Check sheet for the modelled part. Datum: model origin and axes. Units: mm. A direction names the side the tool comes from. Round coordinates to 2 decimals unless told otherwise and drop trailing zeros. Order: outer loops, then holes, each group sorted by start corner. A loop starts at its lowest first (then second) coordinate and runs counter-clockwise, first axis right, second up.
from build123d import *

# Parameters (mm, degrees)
SKETCH1_W           = 30.1625
SKETCH1_H           = 14.2875
BOSS_EXTRUDE1_DEPTH = 6.35
SKETCH2_W           = 30.1625
SKETCH2_H           = 7.9375
BOSS_EXTRUDE2_DEPTH = 6.35
BOSS_EXTRUDE3_DEPTH = 1.5875
SKETCH4_R           = 1.5875
CUT_EXTRUDE1_DEPTH  = 1.5875


with BuildPart() as part:
    # Sketch1 → Boss-Extrude1 (new body)
    with BuildSketch(Plane.XY):
        Rectangle(SKETCH1_W, SKETCH1_H)
    extrude(amount=BOSS_EXTRUDE1_DEPTH)

    # Sketch2 → Boss-Extrude2 (add)
    with BuildSketch(Plane.XY.offset(6.35)):
        Rectangle(SKETCH2_W, SKETCH2_H)
    extrude(amount=BOSS_EXTRUDE2_DEPTH)

    # Sketch3 → Boss-Extrude3 (add)
    with BuildSketch(Plane(origin=(0, 0, 0), x_dir=(-1, 0, 0), z_dir=(0, 0, -1))):
        with BuildLine():
            ThreePointArc((-15.08125, 0), (-16.243669962, 2.806330038), (-19.05, 3.96875))
            Line((-19.05, 3.96875), (-19.05, -3.96875))
            ThreePointArc((-19.05, -3.96875), (-16.243669962, -2.806330038), (-15.08125, 0))
        make_face()
        with BuildLine():
            Line((-19.05, -3.96875), (-19.05, 3.96875))
            ThreePointArc((-19.05, 3.96875), (-23.01875, 0), (-19.05, -3.96875))
        make_face()
        with BuildLine():
            Line((-15.08125, 3.96875), (-19.05, 3.96875))
            ThreePointArc((-19.05, 3.96875), (-16.243669962, 2.806330038), (-15.08125, 0))
            Line((-15.08125, 0), (-15.08125, 3.96875))
        make_face()
        with BuildLine():
            ThreePointArc((-15.08125, 0), (-16.243669962, -2.806330038), (-19.05, -3.96875))
            Line((-19.05, -3.96875), (-15.08125, -3.96875))
            Line((-15.08125, -3.96875), (-15.08125, 0))
        make_face()
    boss_extrude3 = extrude(amount=-BOSS_EXTRUDE3_DEPTH)

    # Sketch4 → Cut-Extrude1 (cut)
    with BuildSketch(Plane.XY.offset(1.5875)):
        with Locations((18.966101938, 0)):
            Circle(SKETCH4_R)
    cut_extrude1 = extrude(amount=-CUT_EXTRUDE1_DEPTH, mode=Mode.SUBTRACT)

    # Mirror1: Boss-Extrude3, Cut-Extrude1 across plane
    add(boss_extrude3.mirror(Plane(origin=(0, 0, 0), x_dir=(0, 0, 1), z_dir=(1, 0, 0))))
    add(cut_extrude1.mirror(Plane(origin=(0, 0, 0), x_dir=(0, 0, 1), z_dir=(1, 0, 0))), mode=Mode.SUBTRACT)


solid = part.part
1) Set-up check for faces 5 (the face through (-17, 3.969, 1)), 6 (the face through (0, -3.969, 9)), 7 (the face through (0, 3.969, 9)): record each of +Z, -Z, +X, -X, +Y, -Y from which the full face is reachable in a straight line by a thin tool's end or side.
2) Gauge pin test, flat ends, axial feed: pin 1 (0.8 mm diameter, centred on x = 18, z = 1, fed in from +Y); pin 2 (4 mm diameter, centred on x = -18.97, y = 0, fed in from +Z); pin 3 (1.7 mm diameter, centred on x = 16, z = 0.5, fed in from -Y). Record the tip position at first contact, or that the pin passes through.
3) Sectioned sample at C-C on z = 11.75. Record the cut outline in (x, y), and give its area (3 significant figures).
4) Sectioned sample at B-B on x = 8. Record the cut outline in (y, z), and give its area (3 significant figures).
5) Sectioned sample at D-D on y = -3. Record the cut outline in (x, z).
6) Sectioned sample at A-A on y = 0. Record the cut outline in (x, z).
7) Scan lines: line 1 (Y direction, x = -5, z = 10.75); line 2 (Z direction, x = 19, y = 2.5); line 3 (X direction, y = -5.5, z = 3). Record each from-to range of solid material in increasing order.
8) Draft check along Y on faces 1 (the face through (-17, -3.969, 1)), 2 (the face through (17, 3.969, 1)), 3 (the face through (-17, 0, 1.588)), 4 (the face through (20.48, 0.48, 0.8)). Enter one of: pulls with the +Y half, pulls with the -Y half, needs draft (parallel to the pull), parting line crosses it, or undercut.
Values found:
1. face 5: +Z, -Z, -X, +Y
1. face 6: +Z, +X, -X, -Y
1. face 7: +Z, +X, -X, +Y
2. pin 1: stops at y = 3.97
2. pin 2: stops at z = 1.59
2. pin 3: stops at y = -3.97
3. outline: (-15.08, -3.97) - (15.08, -3.97) - (15.08, 3.97) - (-15.08, 3.97) - close
3. area: 239 mm2
4. outline: (-7.14, 0) - (7.14, 0) - (7.14, 6.35) - (3.97, 6.35) - (3.97, 12.7) - (-3.97, 12.7) - (-3.97, 6.35) - (-7.14, 6.35) - close
4. area: 141 mm2
5. outline: (-21.65, 0) - (21.65, 0) - (21.65, 1.59) - (15.08, 1.59) - (15.08, 12.7) - (-15.08, 12.7) - (-15.08, 1.59) - (-21.65, 1.59) - close
6. outline: (-23.02, 0) - (-20.55, 0) - (-20.55, 1.59) - (-23.02, 1.59) - close; (-17.38, 0) - (17.38, 0) - (17.38, 1.59) - (15.08, 1.59) - (15.08, 12.7) - (-15.08, 12.7) - (-15.08, 1.59) - (-17.38, 1.59) - close; (20.55, 0) - (23.02, 0) - (23.02, 1.59) - (20.55, 1.59) - close
7. line 1: y = -3.97 to 3.97
7. line 2: z = 0 to 1.59
7. line 3: x = -15.08 to 15.08
8. face 1: pulls with the -Y half
8. face 2: pulls with the +Y half
8. face 3: needs draft
8. face 4: undercut
